Model file for the job. Use its own axes, mm. Give positions to 0.01 mm unless a question says otherwise; leave off trailing zeros. Loops run counter-clockwise (first coordinate to the right, second up) from the corner with the lowest first, then second, coordinate; pieces in that order, holes last. Notation, with made-up numbers: (47, 11) - (78, 11) arc R7 cw to (78, 21) - close; hole circle Ø5 at (31.5, 16.5). An arc over 180 degrees is marked (long way). Use a Markdown table: item, result.
from build123d import *

# Parameters (mm, degrees)
SKETCH1_R           = 101.6
BOSS_EXTRUDE1_DEPTH = 4
CUT_EXTRUDE2_DEPTH  = 144.739764853
CIRPATTERN1_COUNT   = 6
SKETCH5_R           = 4
CUT_EXTRUDE3_DEPTH  = 144.739764853
BOSS_EXTRUDE2_START = 148.4
SKETCH6_R           = 101.6
SKETCH6_R_2         = 100.6
BOSS_EXTRUDE2_DEPTH = 148.4
FILLET1_R           = 2


with BuildPart() as part:
    # Sketch1 → Boss-Extrude1 (new body)
    with BuildSketch(Plane(origin=(0, 0, 0), x_dir=(1, 0, 0), z_dir=(0, 1, 0))):
        with Locations(Location((0, 0, 0), (0, 0, 270))):
            Circle(SKETCH1_R)
    extrude(amount=BOSS_EXTRUDE1_DEPTH)

    # Sketch2 → Cut-Extrude2 (cut, through all)
    with BuildSketch(Plane(origin=(0, 0, 0), x_dir=(1, 0, 0), z_dir=(0, 1, 0))):
        with BuildLine():
            Line((23.571606506, 8.480480962), (75.093958746, 40.675219815))
            ThreePointArc((75.093958746, 40.675219815), (83.497889012, 41.700558349), (89.676425221, 35.912376134))
            ThreePointArc((89.676425221, 35.912376134), (96.6, 0), (89.676425221, -35.912376134))
            ThreePointArc((89.676425221, -35.912376134), (83.497889012, -41.700558349), (75.093958746, -40.675219815))
            Line((75.093958746, -40.675219815), (23.571606506, -8.480480962))
            ThreePointArc((23.571606506, -8.480480962), (18.870799148, 0), (23.571606506, 8.480480962))
        make_face()
    cut_extrude2 = extrude(amount=CUT_EXTRUDE2_DEPTH, mode=Mode.SUBTRACT)

    # CirPattern1: Cut-Extrude2 ×6 about axis
    cirpattern1_axis = Axis((0, 0, 0), (0, 1, 0))
    for i in range(1, CIRPATTERN1_COUNT):
        add(cut_extrude2.rotate(cirpattern1_axis, i * 360 / CIRPATTERN1_COUNT), mode=Mode.SUBTRACT)

    # Sketch5 → Cut-Extrude3 (cut, through all)
    with BuildSketch(Plane(origin=(0, 0, 0), x_dir=(1, 0, 0), z_dir=(0, 1, 0))):
        with Locations(Location((0, 0, 0), (0, 0, 270))):
            Circle(SKETCH5_R)
    extrude(amount=CUT_EXTRUDE3_DEPTH, mode=Mode.SUBTRACT)

    # Sketch6 → Boss-Extrude2 (add)
    with BuildSketch(Plane.XZ.offset(BOSS_EXTRUDE2_START)):
        with Locations(Location((0, 0, 0), (0, 0, 270))):
            Circle(SKETCH6_R)
        with Locations(Location((0, 0, 0), (0, 0, 270))):
            Circle(SKETCH6_R_2, mode=Mode.SUBTRACT)
    extrude(amount=-BOSS_EXTRUDE2_DEPTH)

    # Fillet1
    fillet1_edges = [part.edges().sort_by_distance(p)[0] for p in [
        (0, 0, 100.6),
    ]]
    fillet(fillet1_edges, radius=FILLET1_R)


solid = part.part
(1) Pin check, flat tips, straight feed: P1, Ø1.5, axis at x = 12.5, y = -13, coming from the -Z side; P2, Ø1.5, axis at y = -99.5, z = -67, coming from the -X side; P3, Ø12, axis at x = 8.5, z = -60, coming from the -Y side; P4, Ø9, axis at x = 0, z = 0, coming from the +Y side. Stop position of each tip, or through.
Computed:
| item | result |
|---|---|
| P1 | z = -100.92 |
| P2 | x = -77.03 |
| P3 | y = 0 |
| P4 | y = 4 |
(2) Slice it at B-B, the plane y = -81. Write the cut outline in (x, z), plus the area to 3 significant figures.
Computed:
| item | result |
|---|---|
| outline | circle Ø203.2 at (0, 0); hole circle Ø201.2 at (0, 0) |
| area | 635 mm² |
(3) Slice it at A-A, the plane z = 0. Write the cut outline in (x, y).
Computed:
| item | result |
|---|---|
| outline | (-101.6, -148.4) - (-100.6, -148.4) - (-100.6, -2) arc R2 cw to (-98.6, 0) - (-96.6, 0) - (-96.6, 4) - (-101.6, 4) - close; (-18.87, 0) - (-4, 0) - (-4, 4) - (-18.87, 4) - close; (4, 0) - (18.87, 0) - (18.87, 4) - (4, 4) - close; (96.6, 0) - (98.6, 0) arc R2 cw to (100.6, -2) - (100.6, -148.4) - (101.6, -148.4) - (101.6, 4) - (96.6, 4) - close |
(4) Drill centre lines: probe 1 along X at (y, z) = (2.15, 0); probe 2 along Z at (x, y) = (0, 2); probe 3 along X at (y, z) = (-60, 0). Where is each one in solid material? Low to high. Write a range as [from, to].
Computed:
| item | result |
|---|---|
| probe 1 | [-101.6, -96.6], [-18.87, -4], [4, 18.87], [96.6, 101.6] |
| probe 2 | [-101.6, -4], [4, 101.6] |
| probe 3 | [-101.6, -100.6], [100.6, 101.6] |
